The listing builds one solid part. Answer for the finished solid, in the listing's coordinates (mm). Face numbers are marked on the shaded views. Coordinates: 2 decimals unless noted, no trailing zeros. Use one line per item in the form item = value. Start each with the question number.
Item 1: The mould has two halves that part along Z. Classify the marked faces 1, 2 and 3: released by +Z, released by -Z, zero draft, split by the parting line, or undercut.
Item 2: Consider line 1 along Y through (x, z) = (0, 3.05); line 2 along Y through (x, z) = (0, 4.5); line 3 along X through (y, z) = (0.8, 3). Determine where each line is inside the solid, lowest interval first. Write a range as [from, to].
Item 3: Each of these flat-tipped pins is pushed along its axis until it touches: pin 1 Ø1 at (x, z) = (-1, 5) entering from -Y; pin 2 Ø2 at (y, z) = (2, 2) entering from -X; pin 3 Ø2 at (x, y) = (1, -2) entering from -Z; pin 4 Ø1.5 at (x, z) = (0, 4) entering from -Y. Where does it stop, or does it pass through?
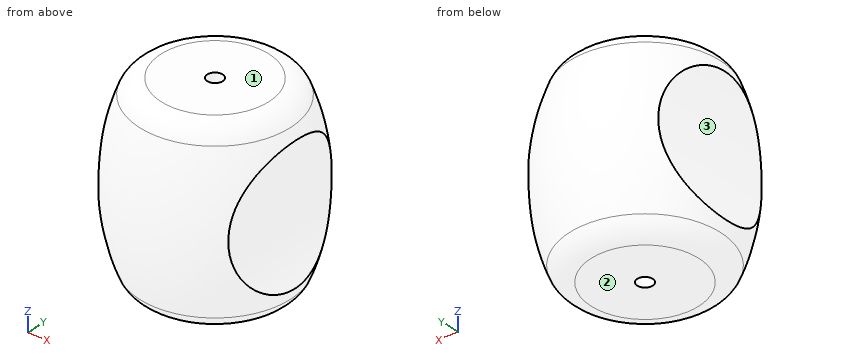
from build123d import *

# Parameters (mm, degrees)
F3_DEPTH      = 3
F3_DEPTH_BACK = 3


with BuildPart() as f1:
    # F0 (on Front) → F1 (revolve)
    with BuildSketch(Plane.XZ):
        with BuildLine():
            Line((0.25, 6), (0.25, 0))
            Line((0.25, 0), (1.75, 0))
            ThreePointArc((1.75, 0), (2.174264, 0.131534), (2.449714, 0.48))
            ThreePointArc((2.449714, 0.48), (2.919048, 3), (2.449714, 5.52))
            ThreePointArc((2.449714, 5.52), (2.174264, 5.868466), (1.75, 6))
            Line((1.75, 6), (0.25, 6))
        make_face()
    revolve(axis=Axis((0, 0, 4.403635), (0, 0, 1)))


with BuildPart() as f3:
    # F2 (on Front) → F3 (new body, two sides)
    with BuildSketch(Plane.XZ) as f3_sk:
        with BuildLine():
            Line((3.75, 5.5), (2.75, 5.5))
            ThreePointArc((2.75, 5.5), (2.080127, 3), (2.75, 0.5))
            Line((2.75, 0.5), (3.75, 0.5))
            Line((3.75, 0.5), (3.75, 5.5))
        make_face()
    extrude(amount=F3_DEPTH)
    extrude(f3_sk.sketch, amount=-F3_DEPTH_BACK)


with BuildPart() as f4_1:
    # F4: instance of F3
    add(f3.part.mirror(Plane.YZ))


with BuildPart() as f1_1:
    add(f1.part)

    # F5: cut F3, F4_1
    add(f3.part, mode=Mode.SUBTRACT)
    add(f4_1.part, mode=Mode.SUBTRACT)


solid = f1_1.part
Response:
q1.face_1 = released by +Z
q1.face_2 = released by -Z
q1.face_3 = undercut
q2.line_1 = [-2.92, -0.25], [0.25, 2.92]
q2.line_2 = [-2.76, -0.25], [0.25, 2.76]
q2.line_3 = [-2.08, 2.08]
q3.pin_1 = -2.64
q3.pin_2 = -2.38
q3.pin_3 = 0
q3.pin_4 = -2.91
